Can you work these out from the model? Positions are in its coordinate system, mm. A direction names the side the tool comes from. Give positions to 0.01 mm unless a question says otherwise; leave off trailing zeros. Order: outer loops, then holes, each group sorted by start corner. A loop starts at its lowest first (then second) coordinate and runs counter-clockwise, first axis right, second up. Notation, with made-up numbers: (28.25, 77.25) - (38.25, 77.25) arc R8 ccw to (38.25, 88.25) - close; hole circle Ø8 at (-23.75, 65). An arc over 180 degrees is marked (long way). Answer as a JSON object with one key per item and string values.
Autodesk Inventor part; units mm, degrees
ref_plane "YZ Plane" through (0, 0, 0) normal (1, 0, 0) x (0, 1, 0)
ref_plane "XZ Plane" through (0, 0, 0) normal (0, 1, 0) x (-1, 0, 0)
ref_plane "XY Plane" through (0, 0, 0) normal (0, 0, 1) x (1, 0, 0)
sketch "Sketch1" plane through (0, 0, 0) normal (0, 1, 0) x (-1, 0, 0)
  line L0 (0, 0) -> (0, -312.648) construction
  line L1 (5, 0) -> (5, -312.648)
  line L2 (-5, -312.648) -> (-5, 0)
  arc A0 (5, 0) -> (-5, 0) centre (0, 0) ccw
  arc A1 (-5, -312.648) -> (5, -312.648) centre (0, -312.648) ccw
  circle A2 centre (0, 0) radius 1.65
  circle A3 centre (0, -312.648) radius 1.65
  circle A4 centre (0, -42.6) radius 1.65
  circle A5 centre (0, -254.274) radius 1.65
  arc A6 (5, -254.274) -> (5, -42.6) centre (-585.5917, -148.437) ccw
  arc A7 (-5, -254.274) -> (-5, -42.6) centre (-595.5917, -148.437) ccw
  point P0 (0, -156.324)
  dimension "d0" = 3.3
  dimension "d1" = 3.3
  dimension "d2" = 10
  dimension "d3" = 312.648
  dimension "d10" = 3.3
  dimension "d11" = 42.6
  dimension "d12" = 3.3
  dimension "d13" = 254.274
  dimension "d16" = 600
  dimension "d17" = 600
extrude "Extrusion1" add sketch "Sketch1" along normal blind 3 contours L1 A1 L2 A7 A0 | A6 L1
sketch "Sketch2" plane through (0, 3, 0) normal (0, 1, 0) x (1, 0, 0)
  line L0 (-83.1437, 348.5388) -> (78.2815, 348.5388)
  line L1 (78.2815, 348.5388) -> (78.2815, -47.0064)
  line L2 (78.2815, -47.0064) -> (-83.1437, -47.0064)
  line L3 (-83.1437, -47.0064) -> (-83.1437, 348.5388)
  line L4 (-31.117, 331.0778) -> (31.6, 331.0778)
  line L5 (31.6, 331.0778) -> (31.6, 150.7662)
  line L6 (31.6, 150.7662) -> (-31.117, 150.7662)
  line L7 (-31.117, 150.7662) -> (-31.117, 331.0778)
  point P0 (0, 0)
extrude "Extrusion2" cut sketch "Sketch2" against normal blind 10
properties part number "Part_5_p2"
Q1. We'd pull the mould along Z, two halves only. Please class faces 3 (the face through (-5, 3, -233)), 4 (the face through (-2.013, 1.479, -201.999)), 5 (the face through (-0.76, 1.48, -252.81)): released by +Z, released by -Z, zero draft, split by the parting line, or undercut.
Recorded:
{"face 3": "zero draft", "face 4": "released by +Z", "face 5": "undercut"}
Q2. If we section it at B-B, the plane x = 0: Please give me the cut outline in (y, z), then the cut area to 3 significant figures.
Recorded:
{"outline": "(0, -317.65) - (3, -317.65) - (3, -314.3) - (0, -314.3) - close; (0, -311) - (3, -311) - (3, -255.92) - (0, -255.92) - close; (0, -252.62) - (3, -252.62) - (3, -221.04) - (0, -221.04) - close", "area": "270 mm^2"}
Q3. I need wall thicknesses on L1, parallel to X at y = 0.4, z = -259; L2, parallel to X at y = 1.95, z = -253.5; L3, parallel to X at y = 1.25, z = -190. Which ranges of each line are inside material? Lowest first, please.
Recorded:
{"L1": "x = -5 to 5", "L2": "x = -5.14 to -1.46, 1.46 to 4.86", "L3": "x = -12.97 to -2.97"}
Q4. If we section it at A-A, the plane y = 1.7: Please give me the cut outline in (x, z), then the cut area to 3 significant figures.
Recorded:
{"outline": "(-14.4, -150.77) arc R600 ccw to (-5, -254.27) - (-5, -312.65) arc R5 ccw to (5, -312.65) - (5, -254.27) arc R600 cw to (-4.4, -150.77) - close; hole circle Ø3.3 at (0, -312.65); hole circle Ø3.3 at (0, -254.27)", "area": "1,640 mm^2"}
Q5. I'm going to push a flat-ended pin straight in: pin 1 Ø1.5 at (y, z) = (1, -279) entering from -X. Where does the tip first touch, or does it pass through?
Recorded:
{"pin 1": "stops at x = -5"}
Q6. If we section it at C-C, the plane z = -222.5: Please give me the cut outline in (x, y).
Recorded:
{"outline": "(-9.82, 0) - (0.18, 0) - (0.18, 3) - (-9.82, 3) - close"}
Q7. Which directions (+Z, -Z, +X, -X, +Y, -Y) give clear straight access to the entire face, cutting with the end or side of a thin tool? Please do faces 1 (the face through (5, 1, -284)), 2 (the face through (-5, 1, -283)).
Recorded:
{"face 1": "+Z, -Z, +X, +Y, -Y", "face 2": "-Z, -X, +Y, -Y"}
